Could you check a few things on this model? Use its own coordinates, in mm. Coordinates: 2 decimals unless noted, no trailing zeros. Loops run counter-clockwise (first coordinate to the right, second up) from the corner with the lowest first, then second, coordinate; pieces in that order, holes last. Notation, with made-up numbers: (-34.75, 71.25) -> (-22.75, 71.25) arc R8 cw to (-22.75, 78.25) -> close; hole circle Ø6 at (-38, 43.5). An arc over 180 degrees is marked (long way). One line per question, with ' | ' between items.
```python
from build123d import *

# Parameters (mm, degrees)
ESQUISSE1_R        = 7
BOSS_EXTRU_1_DEPTH = 8


with BuildPart() as part:
    # Esquisse1 → Boss.-Extru.1 (new body)
    with BuildSketch(Plane(origin=(0, 0, 0), x_dir=(1, 0, 0), z_dir=(0, 1, 0))):
        with BuildLine():
            Line((10, 0), (240, 0))
            ThreePointArc((240, 0), (247.071067812, 2.928932188), (250, 10))
            Line((250, 10), (250, 240))
            ThreePointArc((250, 240), (247.071067812, 247.071067812), (240, 250))
            Line((240, 250), (10, 250))
            ThreePointArc((10, 250), (2.928932188, 247.071067812), (0, 240))
            Line((0, 240), (0, 10))
            ThreePointArc((0, 10), (2.928932188, 2.928932188), (10, 0))
        make_face()
        with Locations(Location((25, 225, 0), (0, 0, 270))):  # turned: the seam where the file's is
            Circle(ESQUISSE1_R, mode=Mode.SUBTRACT)
        with Locations(Location((225, 225, 0), (0, 0, 270))):  # turned: the seam where the file's is
            Circle(ESQUISSE1_R, mode=Mode.SUBTRACT)
        with Locations(Location((225, 25, 0), (0, 0, 270))):  # turned: the seam where the file's is
            Circle(ESQUISSE1_R, mode=Mode.SUBTRACT)
        with Locations(Location((25, 25, 0), (0, 0, 270))):  # turned: the seam where the file's is
            Circle(ESQUISSE1_R, mode=Mode.SUBTRACT)
    extrude(amount=BOSS_EXTRU_1_DEPTH)


solid = part.part
```
Q1. Imagine slicing it at A-A on z = -225. Write out the boundary of the cut face in (x, y), plus the area to 3 significant figures.
Values follow:
outline: (0, 0) -> (18, 0) -> (18, 8) -> (0, 8) -> close; (32, 0) -> (218, 0) -> (218, 8) -> (32, 8) -> close; (232, 0) -> (250, 0) -> (250, 8) -> (232, 8) -> close | area: 1,780 mm2
Q2. For pin 1 (8 mm diameter, centred on x = 97.5, z = -204, fed in from -Y), with a flat end and sliding along its axis, tell me the tip position at first contact or that it passes through.
Values follow:
pin 1: stops at y = 0
Q3. Imagine slicing it at B-B on x = 25. Write out the boundary of the cut face in (y, z).
Values follow:
outline: (0, -250) -> (8, -250) -> (8, -232) -> (0, -232) -> close; (0, -218) -> (8, -218) -> (8, -32) -> (0, -32) -> close; (0, -18) -> (8, -18) -> (8, 0) -> (0, 0) -> close
Q4. Please list where these lines run through material, in increasing order: L1, parallel to X at y = 4.75, z = -225; L2, parallel to X at y = 7.75, z = -219.5; L3, parallel to Z at x = 30.5, y = 1.75. Write a range as [from, to].
Values follow:
L1: x = [0, 18], [32, 218], [232, 250] | L2: x = [0, 20.67], [29.33, 220.67], [229.33, 250] | L3: z = [-250, -229.33], [-220.67, -29.33], [-20.67, 0]
Q5. We'd pull the mould along Z, two halves only. Please class faces 1 (the face through (18.166, 3.944, -26.517)), 2 (the face through (222.319, 3.944, -218.534)), 3 (the face through (2.85, 3.94, -3.01)), 4 (the face through (250, 4, -123)): released by +Z, released by -Z, zero draft, split by the parting line, or undercut.
Values follow:
face 1: undercut | face 2: undercut | face 3: released by +Z | face 4: zero draft
